Check sheet for the modelled part. Datum: model origin and axes. Units: mm. Face numbers are marked on the shaded views. A direction names the side the tool comes from. Coordinates: 2 decimals unless noted, no trailing zeros. Order: outer loops, then holes, each group sorted by start corner. A loop starts at its lowest first (then second) coordinate and runs counter-clockwise, first axis right, second up.
1. Thickness scan on line 1 (Y direction, x = 6, z = 27.55); line 2 (X direction, y = -0.5, z = 1.35); line 3 (Y direction, x = 3, z = 24). Record the ranges inside material, lowest first.
2. Gauge pin test, flat ends, axial feed: pin 1 Ø8 at (x, y) = (15.5, 44) entering from -Z (3 decimals); pin 2 Ø6.5 at (x, z) = (14.5, 25) entering from -Y; pin 3 Ø8.5 at (x, z) = (8, 42) entering from +Y; pin 4 Ø10 at (x, y) = (-11, -1.5) entering from +Z. Record the tip position at first contact, or that the pin passes through.
3. Draft check along Z on the marked faces 5, 6, 7 and 8. Enter one of: released by +Z, released by -Z, zero draft, split by the parting line, or undercut.
4. Cross-section at A-A (y = 27.5). Enter the section's corners in (x, z), then the cut area to 3 significant figures.
5. Cross-section at B-B (x = 20). Count the separate pieces of the cut face and the enclosed holes in it, then the cut area to 3 significant figures.
6. Set-up check for the marked faces 1, 2, 3 and 4: record each of +Z, -Z, +X, -X, +Y, -Y from which the full face is reachable in a straight line by a thin tool's end or side.
7. Cross-section at C-C (y = 13.5). Enter the section's corners in (x, z).
Autodesk Inventor part; units mm, degrees
ref_plane "Plano de trabajo1" through (0, 0, 23) normal (0, 0, 1) x (1, 0, 0)
sketch "Boceto2" plane through (0, 0, 23) normal (0, 0, 1) x (1, 0, 0)
  line L0 (-3, 10) -> (25, 10)
  line L1 (25, 10) -> (25, 65)
  line L2 (23, 67) -> (-1, 67)
  line L3 (-3, 65) -> (-3, 10)
  line L4 (-3, 10) -> (25, 67) construction
  line L5 (25, 10) -> (-3, 67) construction
  line L6 (21.25, 18.406) -> (0.75, 18.406)
  line L7 (0.75, 18.406) -> (0.75, 58.594)
  line L8 (0.75, 58.594) -> (21.25, 58.594)
  line L9 (21.25, 58.594) -> (21.25, 18.406)
  line L10 (21.25, 18.406) -> (0.75, 58.594) construction
  line L11 (0.75, 18.406) -> (21.25, 58.594) construction
  circle A0 centre (6, 63.5) radius 2
  circle A1 centre (16, 63.5) radius 2
  circle A2 centre (6, 13.5) radius 2
  circle A3 centre (16, 13.5) radius 2
  line L12 (25, -6.6) -> (-3, -6.6)
  line L13 (-3, -6.6) -> (-3, 10)
  line L14 (-3, 10) -> (25, 10)
  line L15 (25, 10) -> (25, -6.6)
  line L16 (25, -6.6) -> (-3, 10) construction
  line L17 (-3, -6.6) -> (25, 10) construction
  arc A4 (-1, 67) -> (-3, 65) centre (-1, 65) ccw
  arc A5 (25, 65) -> (23, 67) centre (23, 65) ccw
  point P0 (0, 0)
  point P1 (11, 38.5)
  point P2 (11, 1.7)
  dimension "d5" = 28
  dimension "d6" = 57
  dimension "d9" = 67
  dimension "d10" = 10
  dimension "d12" = 25
  dimension "d13" = 20.5
  dimension "d14" = 40.188
  dimension "d15" = 4
  dimension "d16" = 4
  dimension "d17" = 4
  dimension "d18" = 4
  dimension "d21" = 10
  dimension "d22" = 10
  dimension "d23" = 7
  dimension "d26" = 3.5
  dimension "d27" = 3.5
  dimension "d28" = 3.5
  dimension "d29" = 3.5
  dimension "d38" = 28
  dimension "d39" = 16.6
  dimension "d40" = 25
  dimension "d41" = 10
  dimension "d82" = 2
  dimension "d84" = 7
  dimension "d85" = 9
ref_plane "Plano de trabajo2" through (0, 0, 58) normal (0, 0, 1) x (1, 0, 0)
sketch "Boceto3" plane through (0, 0, 58) normal (0, 0, 1) x (1, 0, 0)
  line L0 (25, 0) -> (-3, 0)
  line L1 (-3, 0) -> (-3, 10)
  line L2 (-3, 10) -> (25, 10)
  line L3 (25, 10) -> (25, 0)
  line L4 (25, 0) -> (-3, 10) construction
  line L5 (-3, 0) -> (25, 10) construction
  point P0 (0, 0)
  point P1 (11, 5)
  dimension "d31" = 28
  dimension "d32" = 10
  dimension "d35" = 10
  dimension "d36" = 25
ref_plane "Plano de trabajo3" through (25, 10, 0) normal (0, 0, 1) x (-1, 0, 0)
sketch "Boceto4" plane through (25, 10, 0) normal (0, 0, 1) x (-1, 0, 0)
  line L0 (0, 0) -> (50, 0)
  line L1 (50, 0) -> (50, 20)
  line L2 (50, 20) -> (0, 20)
  line L3 (0, 20) -> (0, 0)
  line L4 (0, 0) -> (50, 20) construction
  line L5 (50, 0) -> (0, 20) construction
  line L6 (0, 20) -> (0, 0)
  line L7 (28, 0) -> (28, 20)
  point P0 (0, 0)
  dimension "d42" = 50
  dimension "d43" = 20
  dimension "d44" = 50
  dimension "d46" = 28
ref_plane "Plano de trabajo4" through (25, 10, 0) normal (0, 0, 1) x (-1, 0, 0)
sketch "Boceto5" plane through (25, 10, 0) normal (0, 0, 1) x (-1, 0, 0)
  line L0 (28, 0) -> (28, 20)
  line L1 (28, 20) -> (0, 20)
  line L2 (0, 20) -> (0, 0)
  line L3 (0, 0) -> (28, 0)
  point P0 (25, 10)
  dimension "d48" = 20
  dimension "d49" = 28
  dimension "d50" = 20
  dimension "d51" = 28
  dimension "d52" = 25
  dimension "d53" = 10
extrude "Extrusión1" add sketch "Boceto4" along normal blind 3
extrude "Extrusión2" add sketch "Boceto2" along normal blind 6 contours L3 A4 L2 A5 L1 L0
ref_plane "Plano de trabajo5" through (0, 10, 0) normal (0, 1, 0) x (-1, 0, 0)
ref_plane "Plano de trabajo7" through (0, -10, 0) normal (0, 1, 0) x (-1, 0, 0)
loft "Solevación2" add profiles "Boceto3", "Boceto5"
sketch "Boceto9" plane through (0, 10, 0) normal (0, 1, 0) x (-1, 0, 0)
  line L0 (-21.25, 58) -> (-0.75, 58)
  line L1 (-0.75, 58) -> (-0.75, 29)
  line L2 (-0.75, 29) -> (-21.25, 29)
  line L3 (-21.25, 29) -> (-21.25, 58)
  line L4 (-21.25, 58) -> (-0.75, 29) construction
  line L5 (-0.75, 58) -> (-21.25, 29) construction
  line L6 (-23, 29) -> (1, 29)
  line L7 (-25, 58) -> (-25, 29)
  point P0 (0, 0)
  point P1 (-11, 43.5)
  dimension "d91" = 20.5
  dimension "d92" = 29
  dimension "d93" = 29
  dimension "d94" = 3.75
extrude "Extrusión5" add sketch "Boceto9" along normal blind 9
sketch "Boceto10" plane through (0, -10, 0) normal (0, 1, 0) x (-1, 0, 0)
  line L0 (-1, 46) -> (-21, 46)
  line L1 (-21, 46) -> (-21, 3)
  line L2 (-21, 3) -> (-1, 3)
  line L3 (-1, 3) -> (-1, 46)
  line L4 (-1, 46) -> (-21, 3) construction
  line L5 (-21, 46) -> (-1, 3) construction
  line L6 (-25, 58) -> (3, 58)
  line L7 (-25, 58) -> (-25, 3)
  line L8 (3, 58) -> (3, 3)
  line L9 (25, 3) -> (-25, 3)
  point P0 (0, 0)
  point P1 (-11, 24.5)
  dimension "d97" = 20
  dimension "d98" = 43
  dimension "d99" = 12
  dimension "d100" = 4
  dimension "d101" = 4
  dimension "d102" = 0
extrude "Extrusión6" cut sketch "Boceto10" along normal blind 14 contours L3 L2 L1 L0
ref_plane "Plano de trabajo8" through (1, 0, 0) normal (1, 0, 0) x (0, 1, 0)
sketch "Boceto11" plane through (1, 0, 0) normal (1, 0, 0) x (0, 1, 0)
  line L0 (10, 29) -> (24, 29)
  line L1 (24, 29) -> (24, 37)
  line L2 (24, 37) -> (10, 37)
  line L3 (10, 37) -> (10, 29)
  line L4 (10, 29) -> (24, 37) construction
  line L5 (24, 29) -> (10, 37) construction
  line L6 (10, 58) -> (10, 29)
  line L7 (65, 29) -> (10, 29)
  point P0 (0, 0)
  point P1 (17, 33)
  dimension "d106" = 14
  dimension "d107" = 8
  dimension "d108" = 14
  dimension "d109" = 0
extrude "Extrusión7" cut sketch "Boceto11" along normal blind 24 and the other way blind 4
sketch "Boceto12" plane through (-3, 10, 58) normal (0, 1, 0) x (1, 0, 0)
  line L0 (0, 0) -> (0, 21)
  line L1 (3.75, 21) -> (3.75, 0)
  line L2 (3.75, 0) -> (0, 0)
  line L3 (0, 0) -> (0, 21)
  line L4 (35.9308, 19.3547) -> (28, 21)
  line L5 (34.2703, -7.1098) -> (39.6026, 18.5929)
  line L6 (35.9308, 19.3547) -> (39.6026, 18.5929)
  line L7 (39.6026, 18.5929) -> (34.2703, -7.1098)
  line L8 (34.2703, -7.1098) -> (30.5984, -6.348)
  line L9 (3.75, 21) -> (0, 21)
  line L10 (3.75, 21) -> (3.75, 0)
  line L11 (35.9308, 19.3547) -> (30.5984, -6.348)
  line L12 (34.2703, -7.1098) -> (30.5984, -6.348)
  line L13 (3.75, 0) -> (0, 0)
  line L14 (3.75, 21) -> (24.25, 21)
  point P0 (18.3993, 70.2266)
  point P1 (0, 21)
  dimension "d130" = 3.75
  dimension "d131" = 0
extrude "Extrusión9" add sketch "Boceto12" along normal blind 13 contours L0 L9 L1 L2
sketch "Boceto13" plane through (21.25, 10, 58) normal (0, 1, 0) x (1, 0, 0)
  line L0 (3.75, 0) -> (-24.25, 0)
  line L1 (3.75, 0) -> (0, 0)
  line L2 (3.75, 0) -> (-1, 0)
  line L3 (-20.5, 0) -> (0, 0)
  line L4 (-0.25, 12) -> (-0.25, 55)
  line L5 (3.75, 0) -> (3.75, 55)
  line L6 (3.75, 0) -> (-1, 0)
  line L7 (0, 0) -> (3.75, 0)
  line L8 (3.75, 0) -> (3.75, 21)
  line L9 (3.75, 21) -> (0, 21)
  line L10 (0, 21) -> (0, 0)
  line L11 (0, 0) -> (3.75, 21) construction
  line L12 (3.75, 0) -> (0, 21) construction
  point P0 (-21.25, 58)
  point P1 (3.75, 21)
  point P2 (0, 21)
  point P3 (1.875, 10.5)
  dimension "d125" = 3.75
  dimension "d126" = 21
  dimension "d127" = 0
  dimension "d128" = 0
extrude "Extrusión10" add sketch "Boceto13" along normal blind 13
ref_plane "Plano de trabajo9" through (-3, 0, 0) normal (1, 0, 0) x (0, 1, 0)
sketch "Boceto14" plane through (-3, 0, 0) normal (1, 0, 0) x (0, 1, 0)
  line L0 (-4, 54) -> (23, 54)
  line L1 (23, 54) -> (23, 58)
  line L2 (23, 58) -> (-4, 58)
  line L3 (-4, 58) -> (-4, 54)
  line L4 (0, 58) -> (23, 58)
  line L5 (23, 37) -> (23, 58)
  line L6 (10, 37) -> (23, 37)
  point P0 (0, 0)
  dimension "d133" = 0
  dimension "d134" = 4
  dimension "d135" = 0
  dimension "d136" = 27
  dimension "d139" = 17
extrude "Extrusión11" cut sketch "Boceto14" along normal blind 28
ref_plane "Plano de trabajo10" through (0, 0, 54) normal (0, 0, 1) x (1, 0, 0)
sketch "Boceto15" plane through (0, 0, 54) normal (0, 0, 1) x (1, 0, 0)
  line L0 (0.75, 10.0003) -> (21.25, 10.0003)
  line L1 (21.25, 10.0003) -> (21.25, 15.5)
  line L2 (21.25, 15.5) -> (0.75, 15.5)
  line L3 (0.75, 15.5) -> (0.75, 10.0003)
  line L4 (0.75, 18.406) -> (0.75, 58.594)
  line L5 (21.25, 58.594) -> (21.25, 18.406)
  line L6 (0.75, 19) -> (21.25, 19)
  line L7 (25, -0.6897) -> (-3, -0.6897)
  point P0 (0, 0)
  dimension "d141" = 0
  dimension "d142" = 0
  dimension "d143" = 3.5
  dimension "d144" = 10.69
extrude "Extrusión12" cut sketch "Boceto15" against normal blind 20
ref_plane "Plano de trabajo11" through (25, 10, 3) normal (0, 0, 1) x (-1, 0, 0)
sketch "Boceto17" plane through (25, 10, 3) normal (0, 0, 1) x (-1, 0, 0)
  circle A0 centre (37.5, 10.5) radius 1.5
  circle A1 centre (15.5, 10.5) radius 1.5
  line L0 (28, 0) -> (50, 0)
  line L1 (50, 0) -> (50, 20)
  point P0 (25, 10)
  dimension "d154" = 3
  dimension "d155" = 3
  dimension "d156" = 9
  dimension "d157" = 9
  dimension "d158" = 11
  dimension "d159" = 19
hole "Agujero1" at (-12.5, -0.5, 3) direction (0, 0, -1) diameter 3 end through all
hole "Agujero2" at (9.5, -0.5, 3) direction (0, 0, -1) diameter 3 end through all
ref_plane "Plano de trabajo12" through (9.125, 10.0003, 54) normal (0, 0.2588, -0.9659) x (-1, 0, 0)
sketch "Boceto18" plane through (9.125, 10.0003, 54) normal (0, 0.2588, -0.9659) x (-1, 0, 0)
  line L0 (-15.875, -6.4708) -> (-15.875, 46.6551)
  line L1 (16.6517, -12) -> (-15.875, -12)
  line L2 (-15.875, -12) -> (-15.875, 0)
  line L3 (-15.875, 0) -> (16.6517, 0)
  line L4 (16.6517, 0) -> (16.6517, -12)
  line L5 (-12.125, 0) -> (8.375, 0)
  point P0 (9.125, -23.6358)
  dimension "d177" = 12
  dimension "d178" = 0
extrude "Extrusión13" cut sketch "Boceto18" against normal blind 3.5
properties part number "Motor"
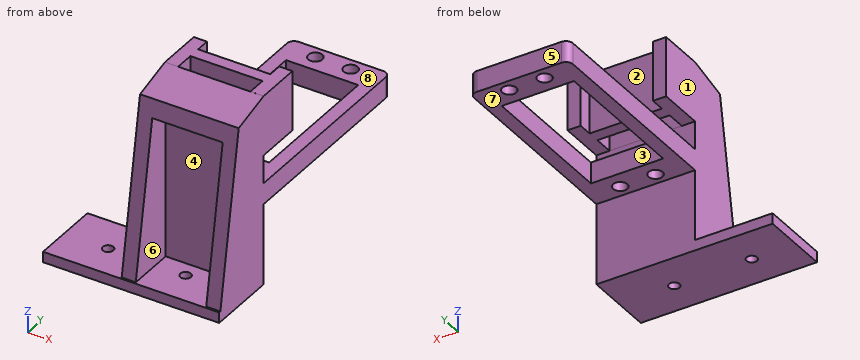
Data:
1. line 1: y = 4 to 11.5, 15.5 to 18.41, 58.59 to 61.5, 65.5 to 67
1. line 2: x = -25 to -14, -11 to 8, 11 to 25
1. line 3: y = 4 to 18.41, 58.59 to 67
2. pin 1: passes through
2. pin 2: stops at y = 4
2. pin 3: stops at y = 19
2. pin 4: stops at z = 3
3. face 5: zero draft
3. face 6: undercut
3. face 7: released by -Z
3. face 8: undercut
4. outline: (-3, 23) - (0.75, 23) - (0.75, 29) - (-3, 29) - close; (21.25, 23) - (25, 23) - (25, 29) - (21.25, 29) - close
4. area: 45.0 mm2
5. separate pieces: 3
5. enclosed holes: 0
5. area: 553 mm2
6. face 1: +Z, -X, +Y, -Y
6. face 2: +Z, -Z, +Y
6. face 3: -Z
6. face 4: -Y
7. outline: (-3, 23) - (4, 23) - (4, 29) - (-3, 29) - close; (-3, 37) - (0.75, 37) - (0.75, 54) - (-3, 54) - close; (8, 23) - (14, 23) - (14, 29) - (8, 29) - close; (18, 23) - (25, 23) - (25, 29) - (18, 29) - close; (21.25, 37) - (25, 37) - (25, 54) - (21.25, 54) - close
